Design review of the part built by this model. Coordinates are the model's own, in mm. Face numbers are marked on the shaded views. A direction names the side the tool comes from. Give positions to 0.01 mm unless a question says otherwise; leave off trailing zeros. Write each loop counter-clockwise with the first axis right and the second up, starting at its lowest first coordinate (ties: lowest second). Pieces come first, ordered by that corner, then holes. Notation, with made-up numbers: M 80.5,8 L 135.5,8 A22 cw 135.5,31 Z; hole C -22,85 d10. An arc over 180 degrees is marked long. Use a Markdown table: item, result. Add a question column.
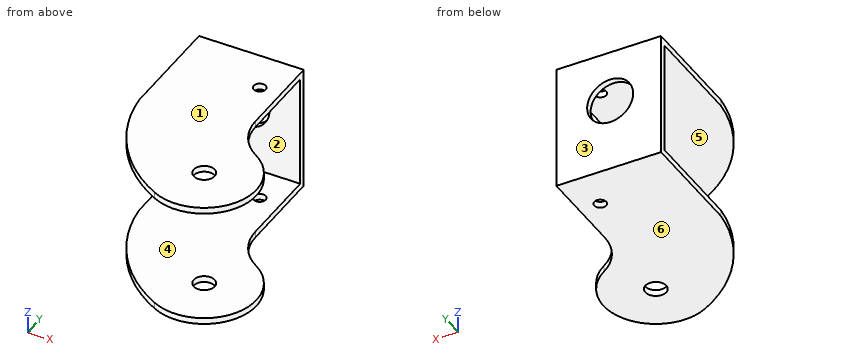
```python
from build123d import *

# Parameters (mm, degrees)
SKETCH_1_R          = 5
SKETCH_1_R_2        = 2.870333843
EXTRUDE_1_DEPTH     = 60
SKETCH_2_W          = 54
SKETCH_2_H          = 139.687150663
CUT_EXTRUDE_1_DEPTH = 74.937741711
SKETCH_3_R          = 11
CUT_EXTRUDE_2_DEPTH = 70


with BuildPart() as part:
    # 草图1 → 凸台-拉伸1 (new body)
    with BuildSketch(Plane.XY):
        with BuildLine():
            Line((-24.281457554, 46.564371273), (-24.281457554, -5.37876517))
            ThreePointArc((-24.281457554, -5.37876517), (-12.44727906, -37.430517799), (13.107980321, -60.108510328))
            ThreePointArc((13.107980321, -60.108510328), (46.43701917, -50.207530875), (37.638484361, -16.570646211))
            ThreePointArc((37.638484361, -16.570646211), (28.903009587, -7.536360283), (25.718542446, 4.620366695))
            Line((25.718542446, 4.620366695), (25.718542446, 46.564371273))
            Line((25.718542446, 46.564371273), (-24.281457554, 46.564371273))
        make_face()
        with Locations((24.656284158, -37.935628727)):
            Circle(SKETCH_1_R, mode=Mode.SUBTRACT)
        with Locations((15.718542446, 26.564371273)):
            Circle(SKETCH_1_R_2, mode=Mode.SUBTRACT)
    extrude(amount=EXTRUDE_1_DEPTH)

    # 草图2 → 切除-拉伸1 (cut, through all)
    with BuildSketch(Plane.ZY.offset(24.281457554)):
        with Locations((30, -26.279204058)):
            Rectangle(SKETCH_2_W, SKETCH_2_H)
    extrude(amount=-CUT_EXTRUDE_1_DEPTH, mode=Mode.SUBTRACT)

    # 草图3 → 切除-拉伸2 (cut)
    with BuildSketch(Plane(origin=(0, 46.564371273, 0), x_dir=(1, 0, 0), z_dir=(0, 1, 0))):
        with Locations((0, -35)):
            Circle(SKETCH_3_R)
    extrude(amount=-CUT_EXTRUDE_2_DEPTH, mode=Mode.SUBTRACT)


solid = part.part
```
(1) Add section B-B on z = 35. Give the boundary of the cut face in (x, y), then the cut area to 3 significant figures.
(2) Add section C-C on x = 6.5. Give the boundary of the cut face in (y, z), then the cut area to 3 significant figures.
(3) Add section D-D on x = -9.5. Give the boundary of the cut face in (y, z).
(4) Add section A-A on y = 32. Give the boundary of the cut face in (x, z).
(5) Wall thickness on L1, parallel to Z at x = 28, y = -33; L2, parallel to X at y = 45, z = 35; L3, parallel to Z at x = 0, y = 44.2: over which ranges is each line inside the solid? List them lowest first.
(6) For pin 1 (6 mm diameter, centred on x = 29.5, y = 16.5, fed in from +Z), flat-tipped, find the tip position at first contact; note if it passes through.
(7) Machinability: for the marked faces 5 and 6, which of the approach directions +Z, -Z, +X, -X, +Y, -Y give a long, thin tool a straight path to every point of the face, cutting with its end or side? Answer none if there is none.
(8) The part is to be moulded in two halves that separate along Z. For the marked faces 1, 2, 3 and 4, say which applies: released by +Z, released by -Z, zero draft, split by the parting line, or undercut.
From the geometry:
| question | item | result |
|---|---|---|
| 1 | outline | M -24.28,43.56 L -11,43.56 L -11,46.56 L -24.28,46.56 Z; M 11,43.56 L 25.72,43.56 L 25.72,46.56 L 11,46.56 Z |
| 1 | area | 84.0 mm^2 |
| 2 | outline | M -56.19,0 L 46.56,0 L 46.56,26.13 L 43.56,26.13 L 43.56,3 L -56.19,3 Z; M -56.19,57 L 43.56,57 L 43.56,43.87 L 46.56,43.87 L 46.56,60 L -56.19,60 Z |
| 2 | area | 725 mm^2 |
| 3 | outline | M -41.43,0 L 46.56,0 L 46.56,29.45 L 43.56,29.45 L 43.56,3 L -41.43,3 Z; M -41.43,57 L 43.56,57 L 43.56,40.55 L 46.56,40.55 L 46.56,60 L -41.43,60 Z |
| 4 | outline | M -24.28,0 L 25.72,0 L 25.72,3 L -24.28,3 Z; M -24.28,57 L 25.72,57 L 25.72,60 L -24.28,60 Z |
| 5 | L1 | z = 0 to 3, 57 to 60 |
| 5 | L2 | x = -24.28 to -11, 11 to 25.72 |
| 5 | L3 | z = 0 to 24, 46 to 60 |
| 6 | pin 1 | passes through |
| 7 | face 5 | +X, -X, -Y |
| 7 | face 6 | -Z, +X, -X, +Y, -Y |
| 8 | face 1 | released by +Z |
| 8 | face 2 | undercut |
| 8 | face 3 | zero draft |
| 8 | face 4 | undercut |
